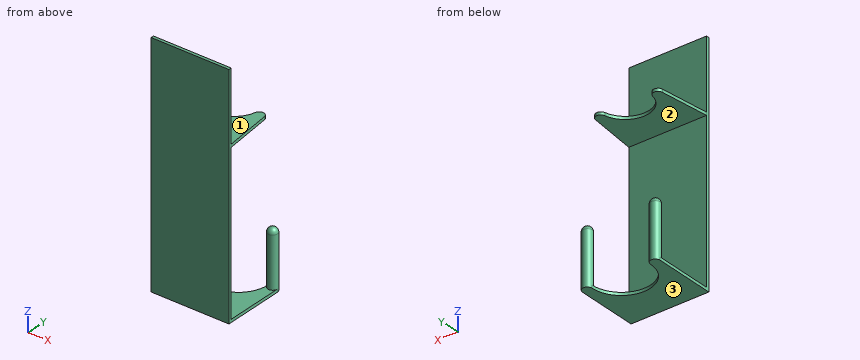
Autodesk Inventor part; units mm, degrees
ref_plane "YZ Plane" through (0, 0, 0) normal (1, 0, 0) x (0, 1, 0)
ref_plane "XZ Plane" through (0, 0, 0) normal (0, 1, 0) x (-1, 0, 0)
ref_plane "XY Plane" through (0, 0, 0) normal (0, 0, 1) x (1, 0, 0)
sketch "Sketch1" plane through (0, 0, 0) normal (0, 0, 1) x (1, 0, 0)
  line L0 (20, 12.5) -> (20, -17.5)
  line L1 (20, -17.5) -> (-20, -17.5)
  line L2 (-20, -17.5) -> (-20, 12.5)
  circle A0 centre (-17.5, 12.5) radius 2.5
  circle A1 centre (17.5, 12.5) radius 2.5
  arc A2 (-15, 12.5) -> (15, 12.5) centre (0, 12.5) ccw
  point P0 (0, 0)
  dimension "d0" = 40
  dimension "d2" = 5
  dimension "d3" = 5
  dimension "d4" = 30
  dimension "d5" = 20
  dimension "d6" = 17.5
  dimension "d7" = 15
extrude "Extrusion1" add sketch "Sketch1" along normal blind 1.5 contours L0 L1 L2 A0 A2 A1
extrude "Extrusion2" add sketch "Sketch1" along normal blind 30 contours A1 | A0
fillet "Fillet1" radius 2.5 2 edges at (-20, 12.5, 30) (15, 12.5, 30)
sketch "Sketch2" plane through (0, 0, 0) normal (0, 0, 1) x (1, 0, 0)
  line L0 (-20, -17.5) -> (20, -17.5)
  line L1 (-20, -17.5) -> (20, -17.5)
  line L2 (-20, -17.5) -> (20, -17.5)
  line L3 (20, -17.5) -> (20, -19)
  line L4 (20, -19) -> (-20, -19)
  line L5 (-20, -19) -> (-20, -17.5)
  point P0 (0, 0)
  dimension "d13" = 1.5
extrude "Extrusion3" add sketch "Sketch2" along normal blind 120
sketch "Sketch5" plane through (-20, -17.5, 1.5) normal (0, 1, 0) x (1, 0, 0)
  line L0 (0, 0) -> (0, -118.5)
  line L1 (40, 0) -> (40, -118.5)
  line L2 (0, -81.0917) -> (40, -81.0917)
  line L3 (40, -81.0917) -> (40, -82.5917)
  line L4 (40, -82.5917) -> (0, -82.5917)
  line L5 (0, -82.5917) -> (0, -81.0917)
  line L6 (0, 0) -> (40, 0)
  point P0 (20, 1.5)
  point P1 (0, -82.5917)
  dimension "d25" = 1.5
  dimension "d26" = 81.0917
extrude "Extrusion5" add sketch "Sketch5" along normal blind 30 contours L2 L1 L4 L0
sketch "Sketch6" plane through (-20, -17.5, 84.0917) normal (0, 0, 1) x (1, 0, 0)
  line L0 (0, 30) -> (0, -1.5)
  line L1 (0, -0.0564) -> (0, 30)
  line L2 (40, 30) -> (0, 30)
  line L3 (0, 30) -> (40, 30)
  line L4 (40, 30) -> (40, -0.0564)
  line L5 (40, -0.0564) -> (0, -0.0564)
  line L6 (0, -0.0564) -> (2.7921, 25.0554)
  arc A0 (7.7306, 25.2572) -> (2.7921, 25.0554) centre (5.2768, 24.7792) ccw
  arc A1 (7.7306, 25.2572) -> (32.2694, 25.2572) centre (20, 27.6473) ccw
  arc A2 (37.2079, 25.0554) -> (32.2694, 25.2572) centre (34.7232, 24.7792) ccw
  line L7 (37.2079, 25.0554) -> (40, -0.0564)
  line L8 (20, -0.0564) -> (20, 30)
  point P0 (20, 17.5)
  dimension "d29" = 2.5
  dimension "d30" = 12.5
  dimension "d31" = 29.4465
  dimension "d32" = 6.344
  dimension "d33" = 30.0564
extrude "Extrusion6" cut sketch "Sketch6" against normal up to surface (1.5 mm away) contours L2 L8 A1 A0 L6 L0 | L2 L4 L7 A2 A1 L8
equation "\"d2\" = arm_thickness"
equation "\"d3\" = arm_thickness"
equation "\"d7\" = 3 * arm_thickness"
equation "\"d8\" = material_thickness"
equation "\"d10\" = arm_length"
equation "\"d12\" = 0.5 * arm_thickness"
equation "\"d13\" = material_thickness"
equation "\"d25\" = material_thickness"
equation "\"d29\" = 0.5 * arm_thickness"
equation "\"arm_thickness\" = 5"
equation "\"material_thickness\" = 1.5"
equation "\"arm_length\" = 30"
properties part number "my_portafilter_holder_§"
Here's how the part is built. I have some questions about the finished solid (model axes, mm). Face numbers are marked on the shaded views. A direction names the side the tool comes from. Coordinates: 2 decimals unless noted, no trailing zeros. Order: outer loops, then holes, each group sorted by start corner. A loop starts at its lowest first (then second) coordinate and runs counter-clockwise, first axis right, second up. Notation, with made-up numbers: M 82.5,12 L 109.5,12 A20 cw 109.5,22 Z; hole C 67.25,-9 d9. An arc over 180 degrees is marked long. Answer as CSV lines item,"result". Start each with the question number.
1. I want a section at B-B, the plane x = 0. Write out the boundary of the cut face in (y, z).
2. I need wall thicknesses on line 1 (Z direction, x = -10, y = 1); line 2 (Y direction, x = -17, z = 37); line 3 (Z direction, x = 12, y = 6). Which ranges of each line are inside material? Lowest first, please. Write a range as [from, to].
3. For pin 1 (1 mm diameter, centred on x = 13.5, y = 5, fed in from +Z); pin 2 (3 mm diameter, centred on x = 11.5, z = 73.5, fed in from +Y); pin 3 (1.5 mm diameter, centred on x = -6, y = 0, fed in from -Z), each with a flat end and sliding along its axis, tell me the tip position at first contact or that it passes through.
4. I want a section at A-A, the plane z = 13.5. Write out the boundary of the cut face in (x, y), and give its area (3 significant figures).
5. I want a section at C-C, the plane y = 1. Write out the boundary of the cut face in (x, z), and give its area (3 significant figures).
6. On a 3-axis mill with a long thin cutter (end or side, diameter ignored), from which of +Z, -Z, +X, -X, +Y, -Y can I reach the whole of each face in a straight line? I mean the marked faces 1, 2 and 3. Say none if no direction works.
7. I want a section at D-D, the plane y = -10. Write out the boundary of the cut face in (x, z), and give its area (3 significant figures).
Recorded:
1,outline,"M -19,0 L -2.5,0 L -2.5,1.5 L -17.5,1.5 L -17.5,82.59 L -2.35,82.59 L -2.35,84.09 L -17.5,84.09 L -17.5,120 L -19,120 Z"
2,line 1,"z = [0, 1.5], [82.59, 84.09]"
2,line 2,"y = [-19, -17.5]"
2,line 3,"z = [82.59, 84.09]"
3,pin 1,"stops at z = 84.09"
3,pin 2,"stops at y = -17.5"
3,pin 3,"stops at z = 82.59"
4,outline,"M -20,-19 L 20,-19 L 20,-17.5 L -20,-17.5 Z; C -17.5,12.5 d5; C 17.5,12.5 d5"
4,area,"99.3 mm2"
5,outline,"M -20,0 L -9.63,0 L -9.63,1.5 L -20,1.5 Z; M -17.94,82.59 L -8.52,82.59 L -8.52,84.09 L -17.94,84.09 Z; M 8.52,82.59 L 17.94,82.59 L 17.94,84.09 L 8.52,84.09 Z; M 9.63,0 L 20,0 L 20,1.5 L 9.63,1.5 Z"
5,area,"59.4 mm2"
6,face 1,"+Z, +X, -X, +Y"
6,face 2,"+X, -X, +Y"
6,face 3,"-Z, +X, -X, +Y, -Y"
7,outline,"M -20,0 L 20,0 L 20,1.5 L -20,1.5 Z; M -19.16,82.59 L 19.16,82.59 L 19.16,84.09 L -19.16,84.09 Z"
7,area,"117 mm2"
